Verification items for this drawing (mm, ordinates from the low corner). A direction names the side the tool comes from. Coordinates: 2 decimals unless noted, no trailing zeros. Loops run counter-clockwise (first coordinate to the right, second up) from the corner with the lowest first, then second, coordinate; pieces in that order, holes last. Notation, with made-up numbers: (32, -25) - (77, -25) arc R19 cw to (77, 1) - close; hole circle Ø2 at (62, -35). An arc over 180 degrees is marked (long way). One line per item, written item: value. Start each with the question number.
(1) Set-up check for the marked faces 1, 2 and 3: record each of +Z, -Z, +X, -X, +Y, -Y from which the full face is reachable in a straight line by a thin tool's end or side.
(2) Section check D-D (y = 14.5). Record the boundary of the cut face in (x, z).
(3) Section check C-C (x = 17.5). Record the boundary of the cut face in (y, z), plus the area to 3 significant figures.
(4) Thickness scan on probe 1 along Z at (x, y) = (4.5, 2.2); probe 2 along Z at (x, y) = (21.5, 23); probe 3 along Z at (x, y) = (25.5, 5). Record the ranges inside material, lowest first. Write a range as [from, to].
(5) Section check A-A (y = 23). Count the separate pieces of the cut face and the enclosed holes in it, plus the area to 3 significant figures.
(6) Draft check along Z on the marked faces 4, 5 and 6. Enter one of: +Z half, -Z half, draft (parallel to the pull), parting line (faces both ways), or undercut.
(7) Section check B-B (z = 19.5). Record the boundary of the cut face in (x, y).
(8) Gauge pin test, flat ends, axial feed: P1, Ø16, axis at x = 17.5, y = 12, coming from the +Z side; P2, Ø5, axis at y = 18.5, z = 21.5, coming from the -X side; P3, Ø10.5, axis at y = 14, z = 44, coming from the +X side. Record the tip position at first contact, or that the pin passes through.
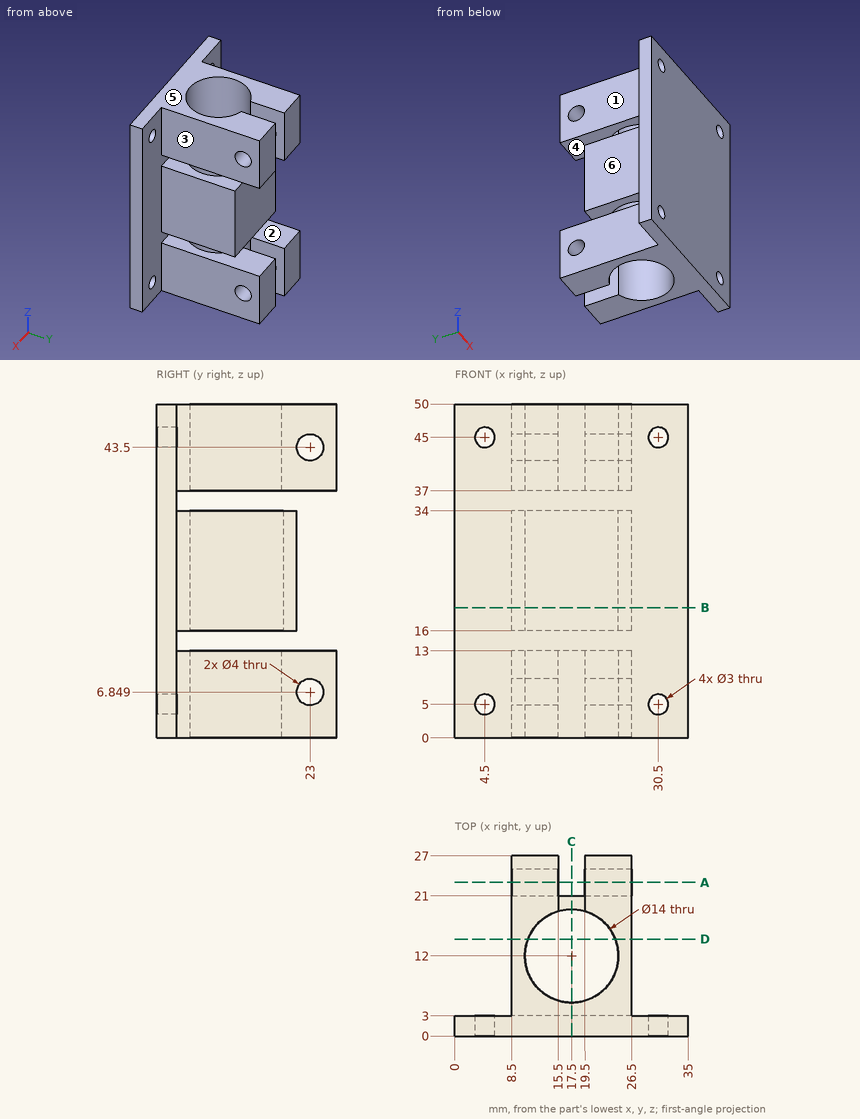
Responses:
1. face 1: +Z, -Z, -X, +Y
1. face 2: +X, -X, +Y
1. face 3: +Z, -Z, +X, +Y
2. outline: (8.5, 0) - (10.96, 0) - (10.96, 13) - (8.5, 13) - close; (8.5, 16) - (10.96, 16) - (10.96, 34) - (8.5, 34) - close; (8.5, 37) - (10.96, 37) - (10.96, 50) - (8.5, 50) - close; (24.04, 0) - (26.5, 0) - (26.5, 13) - (24.04, 13) - close; (24.04, 16) - (26.5, 16) - (26.5, 34) - (24.04, 34) - close; (24.04, 37) - (26.5, 37) - (26.5, 50) - (24.04, 50) - close
3. outline: (0, 0) - (5, 0) - (5, 13) - (3, 13) - (3, 16) - (5, 16) - (5, 34) - (3, 34) - (3, 37) - (5, 37) - (5, 50) - (0, 50) - close; (19, 16) - (21, 16) - (21, 34) - (19, 34) - close
3. area: 274 mm²
4. probe 1: z = [0, 3.5], [6.5, 43.5], [46.5, 50]
4. probe 2: z = [0, 4.85], [8.85, 13], [37, 41.5], [45.5, 50]
4. probe 3: z = [0, 13], [16, 34], [37, 50]
5. separate pieces: 8
5. enclosed holes: 0
5. area: 252 mm²
6. face 4: undercut
6. face 5: +Z half
6. face 6: draft
7. outline: (0, 0) - (35, 0) - (35, 3) - (26.5, 3) - (26.5, 21) - (8.5, 21) - (8.5, 3) - (0, 3) - close; hole circle Ø14 at (17.5, 12)
8. P1: stops at z = 50
8. P2: stops at x = 8.5
8. P3: stops at x = 26.5
